from build123d import *

# Parameters (mm, degrees)
SKETCH_1_W          = 110
SKETCH_1_H          = 120
EXTRUDE_1_DEPTH     = 30
EXTRUDE_2_DEPTH     = 110
SKETCH_3_W          = 40
SKETCH_3_H          = 60
CUT_EXTRUDE_1_DEPTH = 3


with BuildPart() as part:
    # 스케치1 → 보스-돌출1 (new body)
    with BuildSketch(Plane.XY):
        with Locations((-9.053023491, -24.839285714)):
            Rectangle(SKETCH_1_W, SKETCH_1_H)
    extrude(amount=EXTRUDE_1_DEPTH)

    # 스케치2 → 보스-돌출2 (add)
    with BuildSketch(Plane(origin=(45.946976509, 0, 0), x_dir=(0, 0, -1), z_dir=(1, 0, 0))):
        with BuildLine():
            Line((0, 35.160714286), (1, 35.160714286))
            ThreePointArc((1, 35.160714286), (5.949747468, 33.110461754), (8, 28.160714286))
            Line((8, 28.160714286), (8, -77.839285714))
            ThreePointArc((8, -77.839285714), (5.949747468, -82.789033183), (1, -84.839285714))
            Line((1, -84.839285714), (0, -84.839285714))
            Line((0, -84.839285714), (0, 35.160714286))
        make_face()
    extrude(amount=-EXTRUDE_2_DEPTH)

    # 스케치3 → 컷-돌출1 (cut)
    with BuildSketch(Plane(origin=(0, 0, -8), x_dir=(-1, 0, 0), z_dir=(0, 0, -1))):
        with Locations((-15.946976509, -24.839285714)):
            Rectangle(SKETCH_3_W, SKETCH_3_H)
    extrude(amount=-CUT_EXTRUDE_1_DEPTH, mode=Mode.SUBTRACT)


solid = part.part
Verification items for the finished model (mm, model axes). A direction names the side the tool comes from. Give positions to 0.01 mm unless a question says otherwise; leave off trailing zeros. Write each loop counter-clockwise with the first axis right and the second up, starting at its lowest first coordinate (ties: lowest second). Pieces come first, ordered by that corner, then holes.
(1) Gauge pin test, flat ends, axial feed: pin 1 (3.5 mm diameter, centred on x = 10.5, z = -7, fed in from +Y); pin 2 (3.5 mm diameter, centred on x = 25.5, z = -6.5, fed in from -Y); pin 3 (8 mm diameter, centred on x = 35, y = -8, fed in from -Z). Record the tip position at first contact, or that the pin passes through.
(2) Cross-section at B-B (x = 1.5). Enter the section's corners in (y, z).
(3) Access from +Z, -Z, +X, -X, +Y, -Y to the whole of each face (thin tool, end or side, straight path). Record for faces 1 (the face through (16, 5.161, -7)), 2 (the face through (-8.283, -82.734, -6.004)).
(4) Cross-section at A-A (y = -44). Enter the section's corners in (x, z).
(5) Mould release check, pull along X, two halves, no side actions. Record for faces 3 (the face through (45.947, -24, 11)), 4 (the face through (-64.053, -24, 11)), 5 (the face through (16, -24, -5)), 6 (the face through (-8, -24, -8)): +X half, -X half, draft (parallel to the pull), parting line (faces both ways), or undercut.
(6) Material ranges on line 1 (Z direction, x = 21, y = -29.5); line 2 (Z direction, x = -27.5, y = -78.5); line 3 (Y direction, x = 3.5, z = -6), recorded low to high.
Worked out:
1. pin 1: stops at y = 33.72
1. pin 2: stops at y = -83.75
1. pin 3: stops at z = -8
2. outline: (-84.84, -1) arc R7 ccw to (-77.84, -8) - (-54.84, -8) - (-54.84, -5) - (5.16, -5) - (5.16, -8) - (28.16, -8) arc R7 ccw to (35.16, -1) - (35.16, 30) - (-84.84, 30) - close
3. face 1: -Z
3. face 2: -Z, +X, -X, -Y
4. outline: (-64.05, -8) - (-4.05, -8) - (-4.05, -5) - (35.95, -5) - (35.95, -8) - (45.95, -8) - (45.95, 30) - (-64.05, 30) - close
5. face 3: +X half
5. face 4: -X half
5. face 5: undercut
5. face 6: draft
6. line 1: z = -5 to 30
6. line 2: z = -7.97 to 30
6. line 3: y = -82.74 to -54.84, 5.16 to 33.06
